The listing builds one solid part. Answer for the finished solid, in the listing's coordinates (mm). Face numbers are marked on the shaded views. Give positions to 0.01 mm unless a question says otherwise; leave off trailing zeros. Order: outer loops, then holes, each group sorted by start corner. A loop starts at its lowest first (then second) coordinate and runs counter-clockwise, first axis right, second up. Notation, with made-up numbers: (48, 4.25) - (70, 4.25) arc R15 ccw to (70, 32.25) - close; hole circle Ø10 at (-20, 88). An arc over 180 degrees is marked (long way). Answer as CSV lines item,"result". Start each with the question number.
1. Consider line 1 along Z through (x, y) = (2.5, 2.35); line 2 along Y through (x, z) = (-7, 5.75); line 3 along Z through (x, y) = (1, 2.95). Determine where each line is inside the solid, lowest interval first. Write a range as [from, to].
2. Section A-A on z = 4 is taken. Give the vertices of the cut face in (x, y), and give its area (3 significant figures).
3. Flat-ended cylindrical pins translate along their axes: pin 1 (1 mm diameter, centred on x = 12.5, y = 3, fed in from +Z); pin 2 (1 mm diameter, centred on x = -12, z = 2, fed in from +Y). Find the tip coordinate at first contact, or state that the pin passes through.
4. Determine the mould class of the marked faces 1, 2 and 3 for opening direction Z: +Z half, -Z half, draft (parallel to the pull), parting line (faces both ways), or undercut.
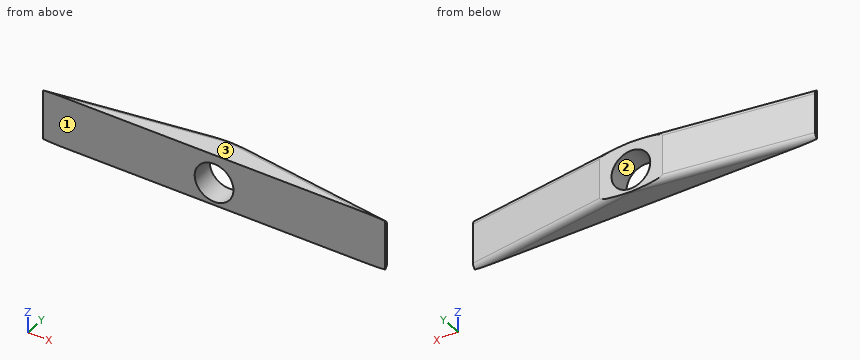
from build123d import *

# Parameters (mm, degrees)
BOSS_EXTRUDE1_DEPTH = 9
SKETCH2_R           = 3.4
CUT_EXTRUDE1_DEPTH  = 32.575306808
FILLET1_R           = 1


with BuildPart() as part:
    # Sketch1 → Boss-Extrude1 (new body)
    with BuildSketch(Plane.XY):
        Polygon((-30, 0), (30, 0), (30, 0.5), (5.5, 4), (-5.5, 4), (-30, 0.5), align=None)
    extrude(amount=BOSS_EXTRUDE1_DEPTH)

    # Sketch2 → Cut-Extrude1 (cut, through all)
    with BuildSketch(Plane(origin=(0, 4, 0), x_dir=(1, 0, 0), z_dir=(0, 1, 0))):
        with Locations(Location((0, -4, 0), (0, 0, 270))):
            Circle(SKETCH2_R)
    extrude(amount=-CUT_EXTRUDE1_DEPTH, mode=Mode.SUBTRACT)

    # Fillet1
    # the kernel refuses this fillet: 1 mm, written as the material it takes off along each edge
    with BuildSketch(Plane(origin=(0.439696962, 4.848528137, 9), x_dir=(0.1414213562373095, -0.9899494936611666, 0), z_dir=(-0.9899494936611666, -0.1414213562373095, 0)), Plane(origin=(35.939696962, -0.348528137, 9), x_dir=(-0.14142135623730948, -0.9899494936611666, 0), z_dir=(-0.9899494936611666, 0.1414213562373095, 0))) as fillet1_piece_1:
        with BuildLine():
            CenterArc((FILLET1_R, -FILLET1_R), FILLET1_R, 90, 90)
            Line((0, -FILLET1_R), (-FILLET1_R * 0.02, -FILLET1_R))
            Line((-FILLET1_R * 0.02, -FILLET1_R), (-FILLET1_R * 0.02, FILLET1_R * 0.02))
            Line((-FILLET1_R * 0.02, FILLET1_R * 0.02), (FILLET1_R, FILLET1_R * 0.02))
            Line((FILLET1_R, FILLET1_R * 0.02), (FILLET1_R, 0))
        make_face()
    extrude(amount=36.748737342, mode=Mode.SUBTRACT)
    with BuildSketch(Plane(origin=(0.439696962, 4.848528137, 0), x_dir=(0.1414213562373095, -0.9899494936611666, 0), z_dir=(-0.9899494936611666, -0.1414213562373095, 0)), Plane(origin=(35.939696962, -0.348528137, 0), x_dir=(-0.14142135623730948, -0.9899494936611666, 0), z_dir=(-0.9899494936611666, 0.1414213562373095, 0))) as fillet1_piece_2:
        with BuildLine():
            CenterArc((FILLET1_R, FILLET1_R), FILLET1_R, 180, 90)
            Line((0, FILLET1_R), (-FILLET1_R * 0.02, FILLET1_R))
            Line((-FILLET1_R * 0.02, FILLET1_R), (-FILLET1_R * 0.02, -FILLET1_R * 0.02))
            Line((-FILLET1_R * 0.02, -FILLET1_R * 0.02), (FILLET1_R, -FILLET1_R * 0.02))
            Line((FILLET1_R, -FILLET1_R * 0.02), (FILLET1_R, 0))
        make_face()
    extrude(amount=36.748737342, mode=Mode.SUBTRACT)


solid = part.part
Checks:
1,line 1,"z = [0, 1.7], [6.3, 9]"
1,line 2,"y = [0, 3.79]"
1,line 3,"z = [0, 0.75], [7.25, 9]"
2,outline,"(-30, 0) - (-3.4, 0) - (-3.4, 4) - (-5.5, 4) - (-30, 0.5) - close; (3.4, 0) - (30, 0) - (30, 0.5) - (5.5, 4) - (3.4, 4) - close"
2,area,"127 mm²"
3,pin 1,"stops at z = 8.87"
3,pin 2,"stops at y = 3.14"
4,face 1,"draft"
4,face 2,"undercut"
4,face 3,"+Z half"
